from build123d import *

# Parameters (mm, degrees)
SKETCH_1_R                = 1.5
EXTRUDE_1_DEPTH           = 3
SKETCH_3_R                = 1.5
EXTRUDE_2_DEPTH           = 7
EXTRUDE_START             = -15.354101966
EXTRUDE_3_DEPTH           = 15.354101966
EXTRUDE_START_2           = -2
EXTRUDE_3_2_DEPTH         = 2
HOLE_WIZARD_1_D           = 3.4
HOLE_WIZARD_1_CSINK_D     = 6.6
HOLE_WIZARD_1_CSINK_ANGLE = 90
CHAMFER_1_SIZE            = 1


with BuildPart() as part:
    # 草图1 → 凸台-拉伸1 (new body)
    with BuildSketch(Plane(origin=(0, 0, 0), x_dir=(1, 0, 0), z_dir=(0, 1, 0))):
        with BuildLine():
            Line((0, 4.5), (12, 4.5))
            Line((12, 4.5), (12, -4.5))
            Line((12, -4.5), (0, -4.5))
            ThreePointArc((0, -4.5), (-4.5, 0), (0, 4.5))
        make_face()
        with Locations(Location((0, 0, 0), (0, 0, 270))):
            Circle(SKETCH_1_R, mode=Mode.SUBTRACT)
    extrude(amount=EXTRUDE_1_DEPTH)

    # 草图3 → 凸台-拉伸2 (add)
    with BuildSketch(Plane(origin=(12, 0, 0), x_dir=(0, 0, -1), z_dir=(1, 0, 0))):
        with BuildLine():
            Line((-4.5, 7.834100358), (-4.5, 0))
            Line((-4.5, 0), (4.5, 0))
            Line((4.5, 0), (4.5, 7.834100358))
            ThreePointArc((4.5, 7.834100358), (0, 12.334100358), (-4.5, 7.834100358))
        make_face()
        with Locations((0, 7.834100358)):
            Circle(SKETCH_3_R, mode=Mode.SUBTRACT)
    extrude(amount=-EXTRUDE_2_DEPTH)

    # 凸台-拉伸3: read off the stored shape, not the designer's step
    # 凸台-拉伸3 outline → 凸台-拉伸3 (add)
    with BuildSketch(Plane(origin=(12, 0, 0), x_dir=(0, 0, -1), z_dir=(1, 0, 0)).offset(EXTRUDE_START)):
        Polygon((-4.5, 0), (-4.5, -1.5), (-3, 0), align=None)
    extrude(amount=EXTRUDE_3_DEPTH)

    # Extrude 3 2 outline → Extrude 3 2 (cut)
    with BuildSketch(Plane(origin=(0, 0, 0), x_dir=(1, 0, 0), z_dir=(0, 1, 0)).offset(EXTRUDE_START_2)):
        with BuildLine():
            Line((-3.354101966, -4.5), (0, -4.5))
            ThreePointArc((0, -4.5), (-1.837117307, -4.107919181), (-3.354101966, -3))
            Line((-3.354101966, -3), (-3.354101966, -4.5))
        make_face()
    extrude(amount=EXTRUDE_3_2_DEPTH, mode=Mode.SUBTRACT)

    # 打孔尺寸(%根据十字)槽半沉头木螺钉的类型1 (through all)
    with Locations(Plane(origin=(0, 3, 0), x_dir=(1, 0, 0), z_dir=(0, 1, 0))):
        with Locations((0, 0)):
            CounterSinkHole(HOLE_WIZARD_1_D / 2, HOLE_WIZARD_1_CSINK_D / 2, counter_sink_angle=HOLE_WIZARD_1_CSINK_ANGLE)

    # 倒角1
    chamfer_1_edges = [part.edges().sort_by_distance(p)[0] for p in [
        (2.5, 3, -4.5),
        (5, 3, 0),
        (5, 12.334100358, 0),
        (5, 5.417050179, -4.5),
        (5, 5.417050179, 4.5),
        (-4.5, 3, 0),
        (2.5, 3, 4.5),
    ]]
    chamfer(chamfer_1_edges, length=CHAMFER_1_SIZE)


solid = part.part
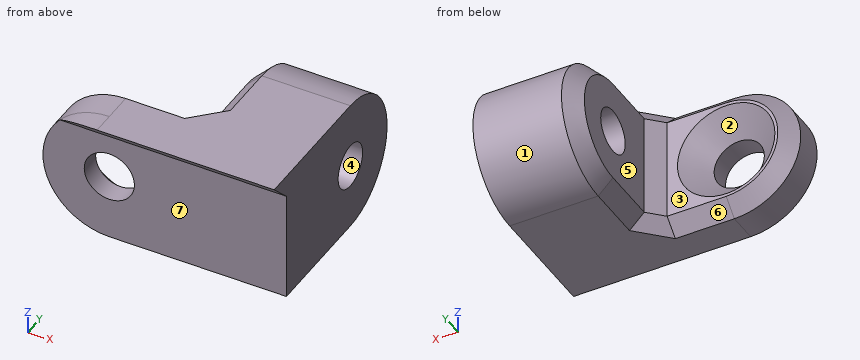
Read the model definition and answer for the solid it produces. Units are mm, in the model's axes. Face numbers are marked on the shaded views. A direction names the side the tool comes from. Round coordinates to 2 decimals unless told otherwise and drop trailing zeros. Write each loop counter-clockwise with the first axis right and the second up, starting at its lowest first coordinate (ties: lowest second). Pieces come first, ordered by that corner, then holes. Notation, with made-up numbers: (1.5, 53.5) - (29.5, 53.5) arc R11 ccw to (29.5, 65.5) - close; hole circle Ø11 at (-9, 3.25). An arc over 180 degrees is marked (long way). Use a Markdown table: item, result.
(1) Straight lines are drawn through the part: line 1 along Y through (x, z) = (8.5, 0); line 2 along X through (y, z) = (2.75, 0.5); line 3 along X through (y, z) = (7, -1.75). For each, find the intervals that lie inside material, in ascending order. Write a range as [from, to].
Reported:
| item | result |
|---|---|
| line 1 | [0, 6.33], [9.33, 12.33] |
| line 2 | [-3.72, -3.01], [3.01, 12] |
| line 3 | [5, 12] |
(2) Which of the six approach directions +Z, -Z, +X, -X, +Y, -Y give full straight-line access (tool end or side, diameter ignored) to the marked faces 5, 6 and 7?
Reported:
| item | result |
|---|---|
| face 5 | +Z, -Z, -X, +Y |
| face 6 | -Z, -X, +Y |
| face 7 | -Z, +X, -X, -Y |
(3) The mould has two halves that part along Z. Classify the marked faces 1, 2, 3 and 4: released by +Z, released by -Z, zero draft, split by the parting line, or undercut.
Reported:
| item | result |
|---|---|
| face 1 | split by the parting line |
| face 2 | undercut |
| face 3 | zero draft |
| face 4 | undercut |
(4) The part is cut by section C-C (y = 2.25). Write down the section's boundary in (x, z), then the cut area to 3 significant figures.
Reported:
| item | result |
|---|---|
| outline | (0, -4.25) - (4, -4.25) - (4.25, -4.5) - (12, -4.5) - (12, 4.5) - (4.25, 4.5) - (4, 4.25) - (0, 4.25) arc R4.25 ccw to start; hole circle Ø5.1 at (0, 0) |
| area | 114 mm2 |
(5) The part is cut by section D-D (y = 7.5). Write down the section's boundary in (x, z), then the cut area to 3 significant figures.
Reported:
| item | result |
|---|---|
| outline | (5, -3.5) - (6, -4.5) - (12, -4.5) - (12, -1.46) - (5, -1.46) - close; (5, 1.46) - (12, 1.46) - (12, 4.5) - (6, 4.5) - (5, 3.5) - close |
| area | 41.5 mm2 |
(6) The part is cut by section B-B (x = 8). Write down the section's boundary in (y, z), then the cut area to 3 significant figures.
Reported:
| item | result |
|---|---|
| outline | (-1.5, 4.5) - (0, 3) - (0, -4.5) - (7.83, -4.5) arc R4.5 ccw to (7.83, 4.5) - close; hole circle Ø3 at (7.83, 0) |
| area | 96.4 mm2 |
(7) The part is cut by section A-A (z = 0). Write down the section's boundary in (x, y).
Reported:
| item | result |
|---|---|
| outline | (-4.5, 0) - (-1.7, 0) - (-1.7, 1.4) - (-3.3, 3) - (-3.5, 3) - (-4.5, 2) - close; (1.7, 0) - (12, 0) - (12, 6.33) - (5, 6.33) - (5, 4) - (4, 3) - (3.3, 3) - (1.7, 1.4) - close; (5, 9.33) - (12, 9.33) - (12, 12.33) - (6, 12.33) - (5, 11.33) - close |
(8) Each of these flat-tipped pins is pushed along its axis until it touches: pin 1 Ø3.5 at (x, z) = (-1, 0) entering from +Y; pin 2 Ø3 at (x, z) = (6.5, 2) entering from -Y; pin 3 Ø2.5 at (x, z) = (0, 0) entering from -Y; pin 4 Ø1.5 at (x, z) = (6.5, -3) entering from +Y. Where does it stop, or does it pass through?
Reported:
| item | result |
|---|---|
| pin 1 | y = 2.45 |
| pin 2 | y = -0.5 |
| pin 3 | through |
| pin 4 | y = 11.73 |
